Geometry check sheet. Reference: the model listing, model coordinates, mm. A direction names the side the tool comes from. Round coordinates to 2 decimals unless told otherwise and drop trailing zeros. Write each loop counter-clockwise with the first axis right and the second up, starting at its lowest first coordinate (ties: lowest second). Pieces come first, ordered by that corner, then holes. Notation, with made-up numbers: (17.25, -23.75) -> (45.25, -23.75) arc R19 ccw to (45.25, -12.75) -> close; hole circle Ø4 at (-36.75, -29). An arc over 180 degrees is marked (long way). Return JSON: item names as keys, results as strings. Group by question number.
from build123d import *

# Parameters (mm, degrees)
ESQUISSE1_W             = 6
ESQUISSE1_H             = 14
ESQUISSE1_R             = 1.5
BOSS_EXTRU_1_DEPTH      = 3
ESQUISSE2_W             = 6
ESQUISSE2_H             = 3
BOSS_EXTRU_2_DEPTH      = 6
ESQUISSE3_R             = 1.5
ENL_V_MAT_EXTRU_1_DEPTH = 10
CHANFREIN3_SIZE         = 1


with BuildPart() as part:
    # Esquisse1 → Boss.-Extru.1 (new body)
    with BuildSketch(Plane.XY):
        with Locations((-1.02739726, -0.01369863)):
            Rectangle(ESQUISSE1_W, ESQUISSE1_H)
        with Locations((-1.02739726, 2.98630137)):
            Circle(ESQUISSE1_R, mode=Mode.SUBTRACT)
    extrude(amount=BOSS_EXTRU_1_DEPTH)

    # Esquisse2 → Boss.-Extru.2 (add)
    with BuildSketch(Plane.XY.offset(3)):
        with Locations((-1.02739726, -5.51369863)):
            Rectangle(ESQUISSE2_W, ESQUISSE2_H)
    extrude(amount=BOSS_EXTRU_2_DEPTH)

    # Esquisse3 → Enlèv. mat.-Extru.1 (cut)
    with BuildSketch(Plane(origin=(0, -7.01369863, 0), x_dir=(-1, 0, 0), z_dir=(0, -1, 0))):
        with Locations(Location((0.52739726, -6, 0), (0, 0, 90))):
            Circle(ESQUISSE3_R)
    extrude(amount=-ENL_V_MAT_EXTRU_1_DEPTH, mode=Mode.SUBTRACT)

    # Chanfrein3
    chanfrein3_edges = [part.edges().sort_by_distance(p)[0] for p in [
        (-2.52739726, 2.98630137, 3),
    ]]
    chamfer(chanfrein3_edges, length=CHANFREIN3_SIZE)


solid = part.part
1) Mould release check, pull along Z, two halves, no side actions. Record for faces 3 (the face through (-1, -7.014, 4)), 4 (the face through (-0.5, -5.5, 7.5)), 5 (the face through (-1, 0, 0)): +Z half, -Z half, draft (parallel to the pull), parting line (faces both ways), or undercut.
2) Sectioned sample at B-B on y = -5. Enter the section's corners in (x, z), and give its area (3 significant figures).
3) Go/stop test with flat-tipped pins: P1, Ø1.8, axis at x = -0.53, z = 6, coming from the +Y side; P2, Ø3, axis at x = -1, z = 5.5, coming from the +Y side. Record where each tip stops, or that it passes through.
4) Tool access check on faces 1 (the face through (-2.4, -4.014, 6)), 2 (the face through (-1, 6.986, 1)). Record the directions out of +Z, -Z, +X, -X, +Y, -Y that give a thin tool (end or side, any length) a straight path to the whole face; none if there is none.
5) Sectioned sample at D-D on z = 4.75. Enter the section's corners in (x, y).
6) Material ranges on probe 1 along Z at (x, y) = (0.45, 0); probe 2 along Y at (x, z) = (-3.25, 3.75); probe 3 along Y at (x, z) = (0.25, 1), recorded low to high. Write a range as [from, to].
7) Sectioned sample at C-C on y = 0. Enter the section's corners in (x, z), and give its area (3 significant figures).
8) Sectioned sample at A-A on z = 6. Enter the section's corners in (x, y), and give its area (3 significant figures).
Evaluation:
{
 "1": {"face 3": "draft", "face 4": "undercut", "face 5": "-Z half"},
 "2": {"outline": "(-4.03, 0) -> (1.97, 0) -> (1.97, 9) -> (-4.03, 9) -> close; hole circle Ø3 at (-0.53, 6)", "area": "46.9 mm2"},
 "3": {"P1": "passes through", "P2": "stops at y = -4.01"},
 "4": {"face 1": "+Z, +X, -X, +Y", "face 2": "+Z, -Z, +X, -X, +Y"},
 "5": {"outline": "(-4.03, -7.01) -> (-1.36, -7.01) -> (-1.36, -4.01) -> (-4.03, -4.01) -> close; (0.3, -7.01) -> (1.97, -7.01) -> (1.97, -4.01) -> (0.3, -4.01) -> close"},
 "6": {"probe 1": "z = [0, 3]", "probe 2": "y = [-7.01, -4.01]", "probe 3": "y = [-7.01, 2.2], [3.77, 6.99]"},
 "7": {"outline": "(-4.03, 0) -> (1.97, 0) -> (1.97, 3) -> (-4.03, 3) -> close", "area": "18.0 mm2"},
 "8": {"outline": "(-4.03, -7.01) -> (-2.03, -7.01) -> (-2.03, -4.01) -> (-4.03, -4.01) -> close; (0.97, -7.01) -> (1.97, -7.01) -> (1.97, -4.01) -> (0.97, -4.01) -> close", "area": "9.00 mm2"}
}
